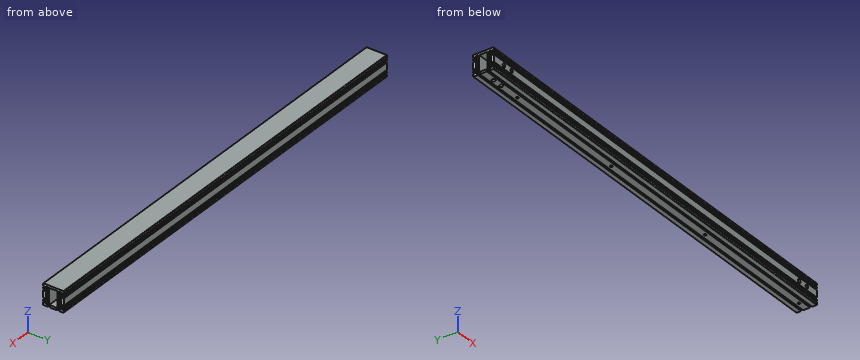
```python
from build123d import *

# Parameters (mm, degrees)
SKETCH_1_W             = 23.5
SKETCH_1_H             = 12
EXTRUDE_1_DEPTH        = 318.5
HOLE_WIZARD_M6_1_D     = 5
HOLE_WIZARD_M6_1_DEPTH = 15
HOLE_WIZARD_M6_1_TIP   = 1.502151548
HOLE_WIZARD_M6_2_D     = 5
HOLE_WIZARD_M6_2_DEPTH = 15
HOLE_WIZARD_M6_2_TIP   = 1.502151548
HOLE_WIZARD_M4_1_D     = 3.3
HOLE_WIZARD_M4_1_DEPTH = 10.1
HOLE_WIZARD_M4_1_TIP   = 0.991420021


with BuildPart() as part:
    # 草图1 → 凸台-拉伸1 (new, symmetric)
    with BuildSketch(Plane(origin=(0, 0, 0), x_dir=(0, 0, -1), z_dir=(1, 0, 0))):
        with BuildLine():
            Line((-14, 15), (-11.5, 15))
            Line((-11.5, 15), (-11.5, 13.5))
            Line((-11.5, 13.5), (-11.4, 13.5))
            ThreePointArc((-11.4, 13.5), (-11.117157288, 13.382842712), (-11, 13.1))
            Line((-11, 13.1), (-11, 12))
            Line((-11, 12), (-9.5, 12))
            Line((-9.5, 12), (-9.5, 15))
            Line((-9.5, 15), (-8, 15))
            Line((-8, 15), (-8, 12.5))
            Line((-8, 12.5), (-5, 12.5))
            Line((-5, 12.5), (-5, 15))
            Line((-5, 15), (5, 15))
            Line((5, 15), (5, 12.5))
            Line((5, 12.5), (8, 12.5))
            Line((8, 12.5), (8, 15))
            Line((8, 15), (9.5, 15))
            Line((9.5, 15), (9.5, 12))
            Line((9.5, 12), (11, 12))
            Line((11, 12), (11, 13.1))
            ThreePointArc((11, 13.1), (11.117157288, 13.382842712), (11.4, 13.5))
            Line((11.4, 13.5), (11.5, 13.5))
            Line((11.5, 13.5), (11.5, 15))
            Line((11.5, 15), (14, 15))
            ThreePointArc((14, 15), (14.707106781, 14.707106781), (15, 14))
            Line((15, 14), (15, 8))
            Line((15, 8), (12.5, 8))
            Line((12.5, 8), (12.5, 5))
            Line((12.5, 5), (15, 5))
            Line((15, 5), (15, -5))
            Line((15, -5), (12.5, -5))
            Line((12.5, -5), (12.5, -8))
            Line((12.5, -8), (15, -8))
            Line((15, -8), (15, -14))
            ThreePointArc((15, -14), (14.707106781, -14.707106781), (14, -15))
            Line((14, -15), (11.5, -15))
            Line((11.5, -15), (11.5, -13.5))
            Line((11.5, -13.5), (11.4, -13.5))
            ThreePointArc((11.4, -13.5), (11.117157288, -13.382842712), (11, -13.1))
            Line((11, -13.1), (11, -12))
            Line((11, -12), (9.5, -12))
            Line((9.5, -12), (9.5, -15))
            Line((9.5, -15), (8, -15))
            Line((8, -15), (8, -12.5))
            Line((8, -12.5), (5, -12.5))
            Line((5, -12.5), (5, -15))
            Line((5, -15), (-5, -15))
            Line((-5, -15), (-5, -12.5))
            Line((-5, -12.5), (-8, -12.5))
            Line((-8, -12.5), (-8, -15))
            Line((-8, -15), (-9.5, -15))
            Line((-9.5, -15), (-9.5, -12))
            Line((-9.5, -12), (-11, -12))
            Line((-11, -12), (-11, -13.1))
            ThreePointArc((-11, -13.1), (-11.117157288, -13.382842712), (-11.4, -13.5))
            Line((-11.4, -13.5), (-11.5, -13.5))
            Line((-11.5, -13.5), (-11.5, -15))
            Line((-11.5, -15), (-14, -15))
            ThreePointArc((-14, -15), (-14.707106781, -14.707106781), (-15, -14))
            Line((-15, -14), (-15, 14))
            ThreePointArc((-15, 14), (-14.707106781, 14.707106781), (-14, 15))
        make_face()
        with BuildLine():
            Line((12, -10.5), (12, -8.5))
            ThreePointArc((12, -8.5), (11.853553391, -8.146446609), (11.5, -8))
            Line((11.5, -8), (-11.5, -8))
            ThreePointArc((-11.5, -8), (-11.853553391, -8.146446609), (-12, -8.5))
            Line((-12, -8.5), (-12, -10.5))
            ThreePointArc((-12, -10.5), (-11.853553391, -10.853553391), (-11.5, -11))
            Line((-11.5, -11), (11.5, -11))
            ThreePointArc((11.5, -11), (11.853553391, -10.853553391), (12, -10.5))
        make_face(mode=Mode.SUBTRACT)
        with BuildLine():
            Line((-11.5, 11), (11.5, 11))
            ThreePointArc((11.5, 11), (11.853553391, 10.853553391), (12, 10.5))
            Line((12, 10.5), (12, 8.5))
            ThreePointArc((12, 8.5), (11.853553391, 8.146446609), (11.5, 8))
            Line((11.5, 8), (-11.5, 8))
            ThreePointArc((-11.5, 8), (-11.853553391, 8.146446609), (-12, 8.5))
            Line((-12, 8.5), (-12, 10.5))
            ThreePointArc((-12, 10.5), (-11.853553391, 10.853553391), (-11.5, 11))
        make_face(mode=Mode.SUBTRACT)
        Rectangle(SKETCH_1_W, SKETCH_1_H, mode=Mode.SUBTRACT)
    extrude(amount=EXTRUDE_1_DEPTH, both=True)

    # M6 螺纹孔1
    with Locations(Plane(origin=(0, 0, -15), x_dir=(-1, 0, 0), z_dir=(0, 0, -1))):
        with Locations((298.5, -0.143680977), (283.5, 0)):
            Hole(HOLE_WIZARD_M6_1_D / 2, depth=HOLE_WIZARD_M6_1_DEPTH)
            with Locations((0, 0, -(HOLE_WIZARD_M6_1_DEPTH + HOLE_WIZARD_M6_1_TIP / 2))):  # 118° drill point
                Cone(0, HOLE_WIZARD_M6_1_D / 2, HOLE_WIZARD_M6_1_TIP, mode=Mode.SUBTRACT)

    # M6 螺纹孔2
    with Locations(Plane.XZ.offset(15)):
        with Locations((-298.5, 0), (-283.5, 0), (283.5, 0), (298.5, 0)):
            Hole(HOLE_WIZARD_M6_2_D / 2, depth=HOLE_WIZARD_M6_2_DEPTH)
            with Locations((0, 0, -(HOLE_WIZARD_M6_2_DEPTH + HOLE_WIZARD_M6_2_TIP / 2))):  # 118° drill point
                Cone(0, HOLE_WIZARD_M6_2_D / 2, HOLE_WIZARD_M6_2_TIP, mode=Mode.SUBTRACT)

    # M4 螺纹孔1
    with Locations(Plane(origin=(0, 0, -15), x_dir=(-1, 0, 0), z_dir=(0, 0, -1))):
        with Locations((-303.5, 0), (-118.5, 0), (66.5, 0), (251.5, 0)):
            Hole(HOLE_WIZARD_M4_1_D / 2, depth=HOLE_WIZARD_M4_1_DEPTH)
            with Locations((0, 0, -(HOLE_WIZARD_M4_1_DEPTH + HOLE_WIZARD_M4_1_TIP / 2))):  # 118° drill point
                Cone(0, HOLE_WIZARD_M4_1_D / 2, HOLE_WIZARD_M4_1_TIP, mode=Mode.SUBTRACT)


solid = part.part
```
CAD build for the part. Positions are in the model's coordinates, mm. Round coordinates to 2 decimals unless told otherwise and drop trailing zeros. Write item = value, one per line. Start each with the question number.
Q1. Drop flat-ended pins along their axis: pin 1 (2 mm diameter, centred on x = -251.5, y = 0, fed in from -Z); pin 2 (0.8 mm diameter, centred on x = -66, z = 10.5, fed in from +Y). Give the stop position or say it passes through.
Q2. Band-saw the part on A-A (x = -164.5). Count the separate pieces of the cut face and the enclosed holes in it, then the cut area to 3 significant figures.
Q3. Probe L1, parallel to Z at x = -198, y = 13.25; L2, parallel to Y at x = -40, z = 0.25; L3, parallel to Y at x = -127.5, z = -13.25. List the from-to ranges inside material, lowest first. Write a range as from..to.
Answers below:
q1.pin_1 = 11.75
q1.pin_2 = 12
q2.separate_pieces = 1
q2.enclosed_holes = 3
q2.area = 407 mm2
q3.L1 = -15..-11.03, -9.5..-8, -5..5, 8..9.5, 11.03..15
q3.L2 = -15..-11, -8..-6, 6..8, 11..15
q3.L3 = -15..-8, -5..5, 8..15
